from build123d import *

# Parameters (mm, degrees)
MOTOR_MOUNT_SOLID_DEPTH              = 7.5
ENCODER_DISTANCE_SKETCH_W            = 50
ENCODER_DISTANCE_SKETCH_H            = 55
ENCODER_DISTANCE_SOLID_DEPTH         = 5
ENCODER_MOUNT_SKETCH_R               = 1.9
ENCODER_MOUNT_SKETCH_W               = 7
ENCODER_MOUNT_SKETCH_H               = 9
ENCODER_MOUNT_SOLID_DEPTH            = 5
MOTOR_CLAMP_MOUNTING_HOLES_SKETCH_R  = 1.9
MOTOR_CLAMP_MOUNTING_HOLES_CUT_DEPTH = 16
GUSSET_PLATE_SKETCH_W                = 50
GUSSET_PLATE_SKETCH_H                = 5
GUSSET_PLATE_SOLID_DEPTH             = 16.5
GUSSET_SOLID_DEPTH                   = 1.5
MOUNTING_PLATE_SKETCH_W              = 50
MOUNTING_PLATE_SKETCH_H              = 92
MOUNTING_PLATE_SKETCH_R              = 2.65
MOUNTING_PLATE_SOLID_DEPTH           = 5
MOUNTING_HOLES_CUT_DEPTH             = 100.036609393
MOUNTING_HOLES_CUT_DEPTH_BACK        = 100.036609393
MOUNTING_HOLE_SKETCH_R               = 2.65
MOUNTING_PLATE_TRIM_SKETCH_W         = 50
MOUNTING_PLATE_TRIM_SKETCH_H         = 15.5
MOUNTING_PLATE_TRIM_SKETCH_H_2       = 40
MOUNTING_PLATE_TRIM_SKETCH_W_2       = 23.5
MOUNTING_PLATE_TRIM_SKETCH_H_3       = 16.5
MOUNTING_PLATE_TRIM_CUT_DEPTH        = 2
CUT_EXTRUDE1_DEPTH                   = 105.216121594
CUT_EXTRUDE1_DEPTH_BACK              = 105.216121594
SKETCH1_W                            = 92
SKETCH1_H                            = 35
SKETCH2_W                            = 50
SKETCH2_H                            = 104.056390977
BOSS_EXTRUDE1_DEPTH                  = 3
SKETCH3_W                            = 8
SKETCH3_H                            = 40
BOSS_EXTRUDE2_DEPTH                  = 25
BOSS_EXTRUDE3_DEPTH                  = 40
CUT_EXTRUDE2_DEPTH                   = 89.489769297
CUT_EXTRUDE2_DEPTH_BACK              = 89.489769297
SKETCH5_R                            = 1.65
CUT_EXTRUDE3_DEPTH                   = 89.489769297
CUT_EXTRUDE3_DEPTH_BACK              = 89.489769297
BOSS_EXTRUDE4_DEPTH                  = 10


with BuildPart() as part:
    # Mouting Mount Sketch → Motor Mount Solid (new, symmetric)
    with BuildSketch(Plane.XY):
        with BuildLine():
            Line((-25, -55), (25, -55))
            Line((25, -55), (25, 0))
            Line((25, 0), (10, 0))
            ThreePointArc((10, 0), (0, -10), (-10, 0))
            Line((-10, 0), (-25, 0))
            Line((-25, 0), (-25, -55))
        make_face()
    extrude(amount=MOTOR_MOUNT_SOLID_DEPTH, both=True)

    # Encoder Distance Sketch → Encoder Distance Solid (add)
    with BuildSketch(Plane.XZ.offset(55)):
        with Locations((0, 20)):
            Rectangle(ENCODER_DISTANCE_SKETCH_W, ENCODER_DISTANCE_SKETCH_H)
    extrude(amount=ENCODER_DISTANCE_SOLID_DEPTH)

    # Encoder Mount Sketch → Encoder Mount Solid (add)
    with BuildSketch(Plane.XY.offset(47.5)):
        Polygon((-25, -60), (-25, -55), (-11.5, 11.5), (11.5, 11.5), (25, -55), (25, -60), align=None)
        with Locations((-8, 8)):
            Circle(ENCODER_MOUNT_SKETCH_R, mode=Mode.SUBTRACT)
        with Locations((8, 8)):
            Circle(ENCODER_MOUNT_SKETCH_R, mode=Mode.SUBTRACT)
        with Locations((-8, -8)):
            Circle(ENCODER_MOUNT_SKETCH_R, mode=Mode.SUBTRACT)
        with Locations((8, -8)):
            Circle(ENCODER_MOUNT_SKETCH_R, mode=Mode.SUBTRACT)
        with Locations((-8, 0)):
            Rectangle(ENCODER_MOUNT_SKETCH_W, ENCODER_MOUNT_SKETCH_H, mode=Mode.SUBTRACT)
        with Locations((8, 0)):
            Rectangle(ENCODER_MOUNT_SKETCH_W, ENCODER_MOUNT_SKETCH_H, mode=Mode.SUBTRACT)
    extrude(amount=ENCODER_MOUNT_SOLID_DEPTH)

    # Motor Clamp Mounting Holes Sketch → Motor Clamp Mounting Holes Cut (cut)
    with BuildSketch(Plane(origin=(0, 0, 0), x_dir=(1, 0, 0), z_dir=(0, 1, 0))):
        with Locations(Location((-15, 0, 0), (0, 0, 180))):
            Circle(MOTOR_CLAMP_MOUNTING_HOLES_SKETCH_R)
        with Locations(Location((15, 0, 0), (0, 0, 180))):
            Circle(MOTOR_CLAMP_MOUNTING_HOLES_SKETCH_R)
    extrude(amount=-MOTOR_CLAMP_MOUNTING_HOLES_CUT_DEPTH, mode=Mode.SUBTRACT)

    # Gusset Plate Sketch → Gusset Plate Solid (add)
    with BuildSketch(Plane.XY.offset(52.5)):
        with Locations((0, -57.5)):
            Rectangle(GUSSET_PLATE_SKETCH_W, GUSSET_PLATE_SKETCH_H)
    extrude(amount=GUSSET_PLATE_SOLID_DEPTH)

    # Gusset Sketch → Gusset Solid (add, symmetric)
    with BuildSketch(Plane(origin=(0, 0, 0), x_dir=(0, 0, -1), z_dir=(1, 0, 0))):
        Polygon((-52.5, 11.5), (-69, -55), (-52.5, -55), align=None)
    extrude(amount=GUSSET_SOLID_DEPTH, both=True)

    # Mounting Plate Sketch → Mounting Plate Solid (add)
    with BuildSketch(Plane(origin=(0, -55, 0), x_dir=(1, 0, 0), z_dir=(0, 1, 0))):
        with Locations((0, -23)):
            Rectangle(MOUNTING_PLATE_SKETCH_W, MOUNTING_PLATE_SKETCH_H)
        with Locations((-19, -63)):
            Circle(MOUNTING_PLATE_SKETCH_R, mode=Mode.SUBTRACT)
        with Locations((19, -63)):
            Circle(MOUNTING_PLATE_SKETCH_R, mode=Mode.SUBTRACT)
        with Locations(Location((-19, 17, 0), (0, 0, 270))):
            Circle(MOUNTING_PLATE_SKETCH_R, mode=Mode.SUBTRACT)
        with Locations(Location((19, 17, 0), (0, 0, 270))):
            Circle(MOUNTING_PLATE_SKETCH_R, mode=Mode.SUBTRACT)
    extrude(amount=-MOUNTING_PLATE_SOLID_DEPTH)

    # Mounting Hole Sketch → Mounting Holes Cut (cut, two sides: drawn at the far end of the back side and taken through both)
    with BuildSketch(Plane(origin=(0, -55, 0), x_dir=(1, 0, 0), z_dir=(0, 1, 0)).offset(-MOUNTING_HOLES_CUT_DEPTH_BACK)):
        with Locations(Location((-19, 17, 0), (0, 0, 270))):
            Circle(MOUNTING_HOLE_SKETCH_R)
        with Locations(Location((19, 17, 0), (0, 0, 270))):
            Circle(MOUNTING_HOLE_SKETCH_R)
        with Locations(Location((19, -63, 0), (0, 0, 90))):
            Circle(MOUNTING_HOLE_SKETCH_R)
        with Locations(Location((-19, -63, 0), (0, 0, 90))):
            Circle(MOUNTING_HOLE_SKETCH_R)
    extrude(amount=MOUNTING_HOLES_CUT_DEPTH + MOUNTING_HOLES_CUT_DEPTH_BACK, mode=Mode.SUBTRACT)

    # Mounting Plate Trim Sketch → Mounting Plate Trim Cut (cut)
    with BuildSketch(Plane(origin=(0, -55, 0), x_dir=(1, 0, 0), z_dir=(0, 1, 0))):
        with Locations((0, 15.25)):
            Rectangle(MOUNTING_PLATE_TRIM_SKETCH_W, MOUNTING_PLATE_TRIM_SKETCH_H)
        with Locations((0, -27.5)):
            Rectangle(MOUNTING_PLATE_TRIM_SKETCH_W, MOUNTING_PLATE_TRIM_SKETCH_H_2)
        with Locations((13.25, -60.75)):
            Rectangle(MOUNTING_PLATE_TRIM_SKETCH_W_2, MOUNTING_PLATE_TRIM_SKETCH_H_3)
        with Locations((-13.25, -60.75)):
            Rectangle(MOUNTING_PLATE_TRIM_SKETCH_W_2, MOUNTING_PLATE_TRIM_SKETCH_H_3)
    extrude(amount=-MOUNTING_PLATE_TRIM_CUT_DEPTH, mode=Mode.SUBTRACT)

    # Sketch1 → Cut-Extrude1 (cut, two sides: drawn at the far end of the back side and taken through both)
    with BuildSketch(Plane.ZY.offset(25).offset(-CUT_EXTRUDE1_DEPTH_BACK)):
        with Locations((23, -42.5)):
            Rectangle(SKETCH1_W, SKETCH1_H)
    extrude(amount=CUT_EXTRUDE1_DEPTH + CUT_EXTRUDE1_DEPTH_BACK, mode=Mode.SUBTRACT)


with BuildPart() as cut_extrude1_piece_1:
    # of the separate pieces the step leaves, piece 1, a body of its own (cut_extrude1_pieces)
    add(part.part.solids().sort_by_distance((-25, -25, -7.5))[0])



with BuildPart() as cut_extrude1_piece_2:
    # of the separate pieces the step leaves, piece 2, a body of its own (cut_extrude1_pieces)
    add(part.part.solids().sort_by_distance((11.5, 11.5, 47.5))[0])


with BuildPart() as cut_extrude1_piece_1_1:
    add(cut_extrude1_piece_1.part)

    add(cut_extrude1_piece_2.part)  # Boss-Extrude1 merges Cut-Extrude1 piece 2
    # Sketch2 → Boss-Extrude1 (add)
    with BuildSketch(Plane.XZ.offset(25)):
        with Locations((0, 9.528195489)):
            Rectangle(SKETCH2_W, SKETCH2_H)
    extrude(amount=BOSS_EXTRUDE1_DEPTH)

    # Sketch3 → Boss-Extrude2 (add)
    with BuildSketch(Plane(origin=(0, -25, 0), x_dir=(1, 0, 0), z_dir=(0, 1, 0))):
        with Locations((16.5, -27.5)):
            Rectangle(SKETCH3_W, SKETCH3_H)
        with Locations((-16.5, -27.5)):
            Rectangle(SKETCH3_W, SKETCH3_H)
    extrude(amount=BOSS_EXTRUDE2_DEPTH)

    # Sketch4 → Boss-Extrude3 (add)
    with BuildSketch(Plane.XY.offset(47.5)):
        Polygon((-15.5, 41), (-20.5, 0), (-12.5, 0), (-10.5, 41), (-10.5, 49), (-15.5, 49), align=None)
        Polygon((10.5, 49), (10.5, 41), (12.5, 0), (20.5, 0), (15.5, 41), (15.5, 49), align=None)
    extrude(amount=-BOSS_EXTRUDE3_DEPTH)

    # Sketch5 → Cut-Extrude2 (cut, two sides: drawn at the far end of the back side and taken through both)
    with BuildSketch(Plane.ZY.offset(15.5).offset(-CUT_EXTRUDE2_DEPTH_BACK)):
        with Locations((32.5, 45)):
            Circle(SKETCH5_R)
    extrude(amount=CUT_EXTRUDE2_DEPTH + CUT_EXTRUDE2_DEPTH_BACK, mode=Mode.SUBTRACT)

    # Sketch6 → Cut-Extrude3 (cut, two sides: drawn at the far end of the back side and taken through both)
    with BuildSketch(Plane.ZY.offset(15.5).offset(-CUT_EXTRUDE3_DEPTH_BACK)):
        Polygon((36.5, 41), (47.5, 11.5), (52.5, 11.5), (52.5, 49), (36.5, 49), align=None)
        Polygon((7.5, 0), (28.5, 41), (28.5, 49), (7.5, 49), align=None)
    extrude(amount=CUT_EXTRUDE3_DEPTH + CUT_EXTRUDE3_DEPTH_BACK, mode=Mode.SUBTRACT)

    # Sketch7 → Boss-Extrude4 (add)
    with BuildSketch(Plane.XY.offset(52.5)):
        Polygon((-11.5, 11.5), (-19.097560976, 11.5), (-20.5, 0), (-20.5, -25), (-18.909774436, -25), align=None)
        Polygon((11.5, 11.5), (18.909774436, -25), (20.5, -25), (20.5, 0), (19.097560976, 11.5), align=None)
    extrude(amount=-BOSS_EXTRUDE4_DEPTH)


solid = cut_extrude1_piece_1_1.part
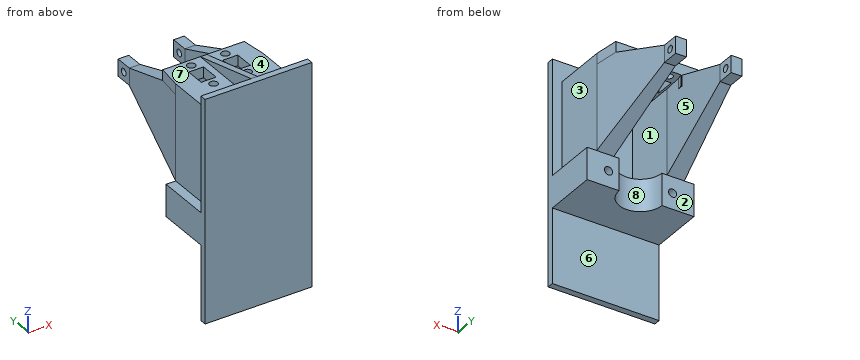
For this review, take the finished solid that the model builds, in its own axes (mm). Face numbers are marked on the shaded views. A direction names the side the tool comes from. Coordinates: 2 decimals unless noted, no trailing zeros. Loops run counter-clockwise (first coordinate to the right, second up) from the corner with the lowest first, then second, coordinate; pieces in that order, holes last. Notation, with made-up numbers: (-36, -37.5) - (-30, -37.5) arc R29 cw to (-30, -11.5) - close; hole circle Ø11 at (4.25, -15.75). An arc over 180 degrees is marked (long way). Use a Markdown table: item, result. Add a question column.
Item 1: We need section D-D (y = -8). Give the number of separate pieces and of enclosed holes in the cut face, and give its area (3 significant figures).
Item 2: Insertion check: pin 1 Ø12 at (x, y) = (-4, 3.5) entering from +Z; pin 2 Ø9 at (y, z) = (46, 31) entering from +X; pin 3 Ø2.5 at (x, y) = (-13.5, 44) entering from +Z. Each pin has a flat end and moves straight along its axis. Give the tip position at first contact, or say it passes through.
Item 3: We need section A-A (x = 8). Give the boundary of the cut face in (y, z).
Item 4: For line 1 (Y direction, x = 8, z = 49); line 2 (X direction, y = 0, z = 35.5); line 3 (Z direction, x = -14, y = 45), list the stretches that pass through material, from the lowest coordinate up.
Item 5: Tool access review of the marked faces 4, 5, 6, 7 and 8: name each direction out of +Z, -Z, +X, -X, +Y, -Y from which nothing blocks a thin tool from reaching the whole face with its end or side.
Item 6: Mouldability with a two-part tool opening along X and no side actions: class the marked faces 1, 2 and 3 as pulls with the +X half, pulls with the -X half, needs draft (parallel to the pull), parting line crosses it, or undercut.
Item 7: We need section C-C (z = 32.5). Give the boundary of the cut face in (x, y).
Item 8: We need section B-B (y = 33). Give the boundary of the cut face in (x, z).
Results list:
| question | item | result |
|---|---|---|
| 1 | separate pieces | 3 |
| 1 | enclosed holes | 2 |
| 1 | area | 1,370 mm^2 |
| 2 | pin 1 | stops at z = 55.84 |
| 2 | pin 2 | stops at x = 15.5 |
| 2 | pin 3 | stops at z = 36.5 |
| 3 | outline | (-28, -42.5) - (-25, -42.5) - (-25, -7.5) - (-6, -7.5) - (-6, 7.5) - (-25, 7.5) - (-25, 47.5) - (-9.9, 47.5) - (-9.9, 52.5) - (-25, 52.5) - (-25, 61.56) - (-28, 61.56) - close; (-6.1, 47.5) - (-4.5, 47.5) - (-4.5, 52.5) - (-6.1, 52.5) - close; (4.5, 47.5) - (6.1, 47.5) - (6.1, 52.5) - (4.5, 52.5) - close; (9.9, 47.5) - (11.5, 47.5) - (11.5, 52.5) - (9.9, 52.5) - close |
| 4 | line 1 | y = -28 to -9.9, -6.1 to -4.5, 4.5 to 6.1, 9.9 to 11.5 |
| 4 | line 2 | x = -20.5 to -12.5, 12.5 to 20.5 |
| 4 | line 3 | z = 28.5 to 30.85, 34.15 to 36.5 |
| 5 | face 4 | +Z, +X, +Y |
| 5 | face 5 | -Z |
| 5 | face 6 | -Z, +X, -X, +Y |
| 5 | face 7 | +Z, -X, +Y |
| 5 | face 8 | -Z, +Y |
| 6 | face 1 | undercut |
| 6 | face 2 | needs draft |
| 6 | face 3 | pulls with the +X half |
| 7 | outline | (-25, -28) - (25, -28) - (25, -25) - (20.5, -25) - (20.5, 0) - (15.5, 41) - (15.5, 43.35) - (10.5, 43.35) - (10.5, 41) - (12.5, 0) - (12.5, -25) - (-12.5, -25) - (-12.5, 0) - (-10.5, 41) - (-10.5, 43.35) - (-15.5, 43.35) - (-15.5, 41) - (-20.5, 0) - (-20.5, -25) - (-25, -25) - close; (-15.5, 46.65) - (-10.5, 46.65) - (-10.5, 49) - (-15.5, 49) - close; (10.5, 46.65) - (15.5, 46.65) - (15.5, 49) - (10.5, 49) - close |
| 8 | outline | (-16.48, 24.4) - (-10.89, 24.4) - (-10.89, 39.48) - (-16.48, 39.48) - close; (10.89, 24.4) - (16.48, 24.4) - (16.48, 39.48) - (10.89, 39.48) - close |
